The model under review builds one solid part; all positions refer to its coordinate system, in mm. Give positions to 0.01 mm unless a question says otherwise; leave off trailing zeros. Write each loop counter-clockwise with the first axis right and the second up, starting at its lowest first coordinate (ties: lowest second). Pieces come first, ordered by that corner, then holes.
from build123d import *

# Parameters (mm, degrees)
F1_R      = 38.4630841236
F2_DEPTH  = 113.792
F2_FACE_R = 38.4630841236
F0_R      = 60.7420219502
F6_R      = 12.7


with BuildPart() as f2:
    # F1 (on face) → F2 (new body)
    with BuildSketch(Plane.XY):
        Circle(F1_R)
    extrude(amount=F2_DEPTH)

    # F2_face (on face) → F3 section 0
    with BuildSketch(Plane.XY.offset(113.792)):
        Circle(F2_FACE_R)
    # F0 (on Top) → F3 section 1
    with BuildSketch(Plane.XY):
        Circle(F0_R)
    loft()

    # F5: F2 across face


with BuildPart() as f2_1:
    add(f2.part)
    add(f2.part.mirror(Plane.XY.offset(113.792)))

    # F6
    f6_edges = [f2_1.edges().sort_by_distance(p)[0] for p in [
        (-60.742022, 0, 227.584),
        (-60.742022, 0, 0),
    ]]
    fillet(f6_edges, radius=F6_R)


solid = f2_1.part
1) Consider section A-A, the plane x = 0. Give the boundary of the cut face in (y, z).
2) To check wall thickness, follow probe 1 along X at (y, z) = (10.5, 182); probe 2 along Y at (x, z) = (31, 176.5); probe 3 along Y at (x, z) = (28.5, 41.5). State the ranges of each line that lie inside material, in increasing order.
3) Insertion check: pin 1 (1 mm diameter, centred on x = -25.5, z = 43.5, fed in from -Y); pin 2 (6 mm diameter, centred on y = -31.5, z = 148, fed in from -X); pin 3 (1 mm diameter, centred on x = -1, z = 97.5, fed in from -Y). Each pin has a flat end and moves straight along its axis. Give the tip position at first contact, or say it passes through.
4) The part is to be moulded in two halves that separate along Z. For faces 1 (the flat face through (-1, 1, 227.584)), 2 (the conical face through (43.98, 13.85, 152.85)), 3 (the flat face through (-1, 1, 0)), say which applies: +Z half, -Z half, draft (parallel to the pull), parting line (faces both ways), or undercut.
5) Consider section C-C, the plane z = 91.5. Give the boundary of the cut face in (x, y), then the cut area to 3 significant figures.
6) Consider section B-B, the plane z = 28. Give the boundary of the cut face in (x, y), then the cut area to 3 significant figures.
Answer block:
1. outline: (-57.78, 15.14) arc R12.7 ccw to (-45.31, 0) - (45.31, 0) arc R12.7 ccw to (57.78, 15.14) - (38.46, 113.79) - (57.78, 212.44) arc R12.7 ccw to (45.31, 227.58) - (-45.31, 227.58) arc R12.7 ccw to (-57.78, 212.44) - (-38.46, 113.79) - close
2. probe 1: x = -50.74 to 50.74
2. probe 2: y = -40.17 to 40.17
2. probe 3: y = -44.23 to 44.23
3. pin 1: stops at y = -45.87
3. pin 2: stops at x = -35.15
3. pin 3: stops at y = -41.74
4. face 1: +Z half
4. face 2: undercut
4. face 3: -Z half
5. outline: circle Ø85.66 at (0, 0)
5. area: 5,760 mm2
6. outline: circle Ø110.52 at (0, 0)
6. area: 9,590 mm2
